Model file for the job. Use its own axes, mm. Face numbers are marked on the shaded views. A direction names the side the tool comes from. Coordinates: 2 decimals unless noted, no trailing zeros. Write each loop counter-clockwise with the first axis right and the second up, starting at its lowest first coordinate (ties: lowest second). Pieces come first, ordered by that corner, then holes.
Q1. Pull direction Y, two halves, no side cores. Call the marked faces 1, 2 and 3: released by +Y, released by -Y, zero draft, split by the parting line, or undercut.
Q2. Band-saw the part on C-C, the plane x = -28.5. Write the cut outline in (y, z).
Q3. Pin check, flat tips, straight feed: P1, Ø4, axis at x = -15.5, y = -46.5, coming from the -Z side; P2, Ø4, axis at x = -9, y = -44.5, coming from the +Z side; P3, Ø5, axis at y = -2, z = 29.5, coming from the +X side. Stop position of each tip, or through.
Q4. Which spindle directions (+Z, -Z, +X, -X, +Y, -Y) get a long thin tool onto all of the face, cutting with end or side? Do the marked faces 4, 5 and 6. Say none if no direction does.
Q5. Band-saw the part on A-A, the plane z = 26. Write the cut outline in (x, y), plus the area to 4 significant figures.
Q6. Band-saw the part on D-D, the plane y = -41. Write the cut outline in (x, z).
Q7. Drill centre lines: probe 1 along Z at (x, y) = (6, 0); probe 2 along Y at (x, z) = (-23, 11); probe 3 along Z at (x, y) = (9, 0). Where is each one in solid material? Low to high.
Q8. Band-saw the part on B-B, the plane y = 0. Write the cut outline in (x, z), plus the area to 3 significant figures.
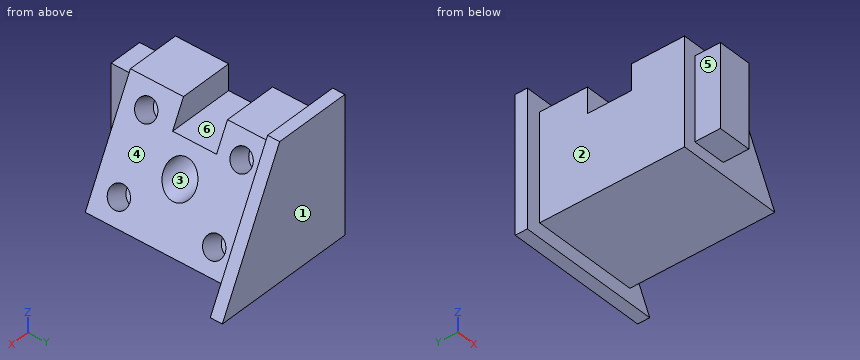
from build123d import *

# Parameters (mm, degrees)
F1_DEPTH  = 38.1
F2_R      = 8.7079162596
F3_DEPTH  = 22.098
F5_DEPTH  = 6.35
F6_R      = 5.7417418986
F7_DEPTH  = 12.954
F8_W      = 23.137550801
F8_H      = 13.5999321938
F9_DEPTH  = 28.448
F10_W     = 17.6125467173
F10_H     = 43.7308948815
F11_DEPTH = 13.462


with BuildPart() as f1:
    # F0 (on Front) → F1 (new body, symmetric)
    with BuildSketch(Plane.XZ):
        Polygon((-26.2284446508, 0), (29.5842699707, 0), (1.6779126599, 56.4308948815), (-26.2284446508, 56.4308948815), align=None)
    extrude(amount=F1_DEPTH, both=True)

    # F2 (on Right) → F3 (cut, symmetric)
    with BuildSketch(Plane.YZ):
        with Locations((0, 27.8683193028)):
            Circle(F2_R)
    extrude(amount=F3_DEPTH, both=True, mode=Mode.SUBTRACT)

    # F4 (on face) → F5 (join)
    with BuildSketch(Plane(origin=(0, 38.1, 0), x_dir=(-1, 0, 0), z_dir=(0, 1, 0))):
        Polygon((33.8484448314, 64.0508950621), (-6.4104854842, 64.0508950621), (-41.8533686003, -7.6200001806), (33.8484448314, -7.6200001806), align=None)
    extrude(amount=F5_DEPTH)

    # F6 (on face) → F7 (cut)
    with BuildSketch(Plane(origin=(23.7710066009, 0, 11.7553018649), x_dir=(0, 1, 0), z_dir=(0.8963824764, 0, 0.4432814636))):
        with Locations((-25.0819269568, 37.4737083912)):
            Circle(F6_R)
        with Locations((25.0819269568, 37.4737083912)):
            Circle(F6_R)
        with Locations((-25.0819269568, -0.7479891615)):
            Circle(F6_R)
        with Locations((25.0819269568, -0.7479891615)):
            Circle(F6_R)
    extrude(amount=-F7_DEPTH, mode=Mode.SUBTRACT)

    # F8 (on Right) → F9 (cut, symmetric)
    with BuildSketch(Plane.YZ):
        with Locations((1.4129802585, 49.6309287846)):
            Rectangle(F8_W, F8_H)
    extrude(amount=F9_DEPTH, both=True, mode=Mode.SUBTRACT)

    # F10 (on face) → F11 (join)
    with BuildSketch(Plane.XZ.offset(38.1)):
        with Locations((-11.0721712921, 28.2154474407)):
            Rectangle(F10_W, F10_H)
    extrude(amount=F11_DEPTH)


solid = f1.part
Answer sheet:
1. face 1: released by +Y
1. face 2: zero draft
1. face 3: undercut
2. outline: (38.1, -7.62) - (44.45, -7.62) - (44.45, 64.05) - (38.1, 64.05) - close
3. P1: stops at z = 6.35
3. P2: stops at z = 50.08
3. P3: stops at x = -22.1
4. face 4: +Z, +X, -Y
4. face 5: +Z, -Z, -X, -Y
4. face 6: +Z, +X, -X
5. outline: (-33.85, 38.1) - (-26.23, 38.1) - (-26.23, -38.1) - (-19.88, -38.1) - (-19.88, -51.56) - (-2.27, -51.56) - (-2.27, -38.1) - (16.73, -38.1) - (16.73, -8.51) - (-22.1, -8.51) - (-22.1, 8.51) - (16.73, 8.51) - (16.73, 38.1) - (25.23, 38.1) - (25.23, 44.45) - (-33.85, 44.45) - close
5. area: 3,225 mm2
6. outline: (-19.88, 6.35) - (-2.27, 6.35) - (-2.27, 50.08) - (-19.88, 50.08) - close
7. probe 1: z = 0 to 19.16, 36.58 to 42.83
7. probe 2: y = -38.1 to 44.45
7. probe 3: z = 0 to 19.16, 36.58 to 41.62
8. outline: (-26.23, 0) - (29.58, 0) - (20.11, 19.16) - (-22.1, 19.16) - (-22.1, 36.58) - (11.5, 36.58) - (8.4, 42.83) - (-26.23, 42.83) - close
8. area: 1,280 mm2
